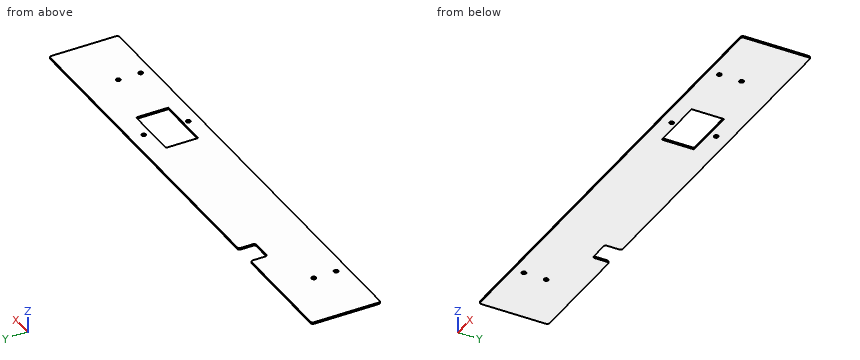
from build123d import *

# Parameters (mm, degrees)
SKETCH1_R           = 1.95
SKETCH1_W           = 49
SKETCH1_H           = 29
BOSS_EXTRUDE1_DEPTH = 1.5
FILLET1_R           = 2
SKETCH3_R           = 1.95
CUT_EXTRUDE1_DEPTH  = 10


with BuildPart() as part:
    # Sketch1 → Boss-Extrude1 (new body)
    with BuildSketch(Plane.XY):
        Polygon((-231.924811832, 29.703517588), (78.075188168, 29.703517588), (78.075188168, -32.296482412), (-351.924811832, -32.296482412), (-351.924811832, 29.703517588), (-251.924811832, 29.703517588), (-251.924811832, 14.703517588), (-231.924811832, 14.703517588), align=None)
        with Locations((-54.924811832, 17.703517588)):
            Circle(SKETCH1_R, mode=Mode.SUBTRACT)
        with Locations((-54.924811832, -22.296482412)):
            Circle(SKETCH1_R, mode=Mode.SUBTRACT)
        with Locations((-54.924811832, -3.296482412)):
            Rectangle(SKETCH1_W, SKETCH1_H, mode=Mode.SUBTRACT)
    extrude(amount=BOSS_EXTRUDE1_DEPTH)

    # Fillet1
    fillet1_edges = [part.edges().sort_by_distance(p)[0] for p in [
        (-351.924811832, 29.703517588, 0.75),
        (-251.924811832, 29.703517588, 0.75),
        (-251.924811832, 14.703517588, 0.75),
        (-231.924811832, 14.703517588, 0.75),
        (-231.924811832, 29.703517588, 0.75),
        (78.075188168, 29.703517588, 0.75),
        (78.075188168, -32.296482412, 0.75),
        (-351.924811832, -32.296482412, 0.75),
    ]]
    fillet(fillet1_edges, radius=FILLET1_R)

    # Sketch3 → Cut-Extrude1 (cut)
    with BuildSketch(Plane(origin=(0, 0, 0), x_dir=(-1, 0, 0), z_dir=(0, 0, -1))):
        with Locations((-23.075188168, -22.296482412)):
            Circle(SKETCH3_R)
        with Locations((-23.075188168, -2.296482412)):
            Circle(SKETCH3_R)
        with Locations((296.924811832, -22.296482412)):
            Circle(SKETCH3_R)
        with Locations((296.924811832, -2.296482412)):
            Circle(SKETCH3_R)
    extrude(amount=-CUT_EXTRUDE1_DEPTH, mode=Mode.SUBTRACT)


solid = part.part
Geometry: final body of the model. Coordinates: model frame, mm. Round coordinates to 2 decimals unless told otherwise and drop trailing zeros. Write each loop counter-clockwise with the first axis right and the second up, starting at its lowest first coordinate (ties: lowest second). Pieces come first, ordered by that corner, then holes. Notation, with made-up numbers: M 16,-20 L 70,-20 A23 cw 70,-8 Z; hole C 18,45.5 d10. An arc over 180 degrees is marked long. Write item = value, one per line.
Item 1: Section query B-B on z = 0.55. Return loops of the section in (x, y).
Findings:
outline = M -351.92,-30.3 A2 ccw -349.92,-32.3 L 76.08,-32.3 A2 ccw 78.08,-30.3 L 78.08,27.7 A2 ccw 76.08,29.7 L -229.92,29.7 A2 ccw -231.92,27.7 L -231.92,16.7 A2 cw -233.92,14.7 L -249.92,14.7 A2 cw -251.92,16.7 L -251.92,27.7 A2 ccw -253.92,29.7 L -349.92,29.7 A2 ccw -351.92,27.7 Z; hole C -296.92,-22.3 d3.9; hole C -296.92,-2.3 d3.9; hole M -79.42,-17.8 L -30.42,-17.8 L -30.42,11.2 L -79.42,11.2 Z; hole C -54.92,-22.3 d3.9; hole C -54.92,17.7 d3.9; hole C 23.08,-22.3 d3.9; hole C 23.08,-2.3 d3.9
Item 2: Section query A-A on y = 6. Return loops of the section in (x, z), then the cut area to 4 significant figures.
Findings:
outline = M -351.92,0 L -79.42,0 L -79.42,1.5 L -351.92,1.5 Z; M -30.42,0 L 78.08,0 L 78.08,1.5 L -30.42,1.5 Z
area = 571.5 mm^2
Item 3: Pin query (flat end, axial travel): P1, Ø3, axis at x = -296.92, y = -22.3, coming from the +Z side. Return the tip coordinate at first contact, or that it passes through.
Findings:
P1 = through
Item 4: Section query C-C on y = 24. Return loops of the section in (x, z).
Findings:
outline = M -351.92,0 L -251.92,0 L -251.92,1.5 L -351.92,1.5 Z; M -231.92,0 L 78.08,0 L 78.08,1.5 L -231.92,1.5 Z
Item 5: Material intervals for line 1 along X through (y, z) = (-2, 1.4); line 2 along X through (y, z) = (27.5, 0.6); line 3 along X through (y, z) = (17, 0.8), sorted ascending. Write a range as [from, to].
Findings:
line_1 = [-351.92, -298.85], [-295, -79.42], [-30.42, 21.15], [25, 78.08]
line_2 = [-351.92, -251.92], [-231.92, 78.08]
line_3 = [-351.92, -251.92], [-231.92, -56.74], [-53.11, 78.08]
